from build123d import *

# Parameters (mm, degrees)
F0_W     = 40
F0_H     = 10
F1_DEPTH = 5
F3_DEPTH = 2.5
F4_R     = 3.5
F5_DEPTH = 7.501
F6_W     = 36.25
F6_H     = 7
F7_DEPTH = 7.501


with BuildPart() as f1:
    # F0 (on Top) → F1 (new body)
    with BuildSketch(Plane.XY):
        with Locations((20, 5)):
            Rectangle(F0_W, F0_H)
    extrude(amount=F1_DEPTH)

    # F2 (on face) → F3 (join)
    with BuildSketch(Plane.XY.offset(5)):
        with BuildLine():
            Line((40, 0), (45, 0))
            ThreePointArc((45, 0), (50, 5), (45, 10))
            Line((45, 10), (40, 10))
            Line((40, 10), (0, 10))
            Line((0, 10), (0, 0))
            Line((0, 0), (40, 0))
        make_face()
    extrude(amount=F3_DEPTH)

    # F4 (on face) → F5 (cut, through all)
    with BuildSketch(Plane.XY.offset(7.5)):
        with Locations((45, 5)):
            Circle(F4_R)
    extrude(amount=-F5_DEPTH, mode=Mode.SUBTRACT)

    # F6 (on face) → F7 (cut, through all)
    with BuildSketch(Plane.XY.offset(7.5)):
        with Locations((19.625, 5)):
            Rectangle(F6_W, F6_H)
    extrude(amount=-F7_DEPTH, mode=Mode.SUBTRACT)

    # F8: F1 across plane


with BuildPart() as f1_1:
    add(f1.part)
    add(f1.part.mirror(Plane.XY))


solid = f1_1.part
Geometry: final body of the model. Coordinates: model frame, mm. A direction names the side the tool comes from. Coordinates: 2 decimals unless noted, no trailing zeros. Order: outer loops, then holes, each group sorted by start corner. A loop starts at its lowest first (then second) coordinate and runs counter-clockwise, first axis right, second up. Notation, with made-up numbers: M 56,15.5 L 111,15.5 A9 cw 111,19.5 Z; hole C 21.25,77 d4. An arc over 180 degrees is marked long. One line per question, with ' | ' between items. Start each with the question number.
Item 1: Draft query along X for faces 1 (the flat face through (41.6, 7.3, -5)), 2 (the flat face through (37.75, 5, 0)), 3 (the flat face through (0, 5, 0)). Return one class per face: released by +X, released by -X, zero draft, split by the parting line, or undercut.
Item 2: Cut plane A-A, the plane z = -2. Return the cut outline in (x, y), then the cut area to 3 significant figures.
Item 3: Pin query (flat end, axial travel): pin 1 Ø5 at (y, z) = (8, -1.5) entering from +X. Return the tip coordinate at first contact, or that it passes through.
Item 4: Cut plane D-D, the plane z = 6.5. Return the cut outline in (x, y).
Item 5: Cut plane B-B, the plane y = 5. Return the cut outline in (x, z), then the cut area to 4 significant figures.
Item 6: Cut plane C-C, the plane x = 22. Return the cut outline in (y, z), then the cut area to 3 significant figures.
Item 7: Ray query, probe 1 along Y at (x, z) = (33, 2); probe 2 along X at (y, z) = (5.5, -2); probe 3 along Z at (x, y) = (40.5, 1.75). Return the intervals inside material, ascending. Write a range as [from, to].
Item 8: Set-up query: faces 4 (the flat face through (41.6, 7.3, 5)), 5 (the flat face through (27, 9, -7.5)), 6 (the flat face through (19, 1.5, 0)). Return all of +Z, -Z, +X, -X, +Y, -Y with unobstructed straight access to the full face (end or side cutting, diameter ignored); none if empty.
A:
1) face 1: zero draft | face 2: undercut | face 3: released by -X
2) outline: M 0,0 L 40,0 L 40,10 L 0,10 Z; hole M 1.5,1.5 L 37.75,1.5 L 37.75,8.5 L 1.5,8.5 Z | area: 146 mm2
3) pin 1: stops at x = 40
4) outline: M 0,0 L 45,0 A5 ccw 45,10 L 0,10 Z; hole M 1.5,1.5 L 37.75,1.5 L 37.75,8.5 L 1.5,8.5 Z; hole C 45,5 d7
5) outline: M 0,-7.5 L 1.5,-7.5 L 1.5,7.5 L 0,7.5 Z; M 37.75,-7.5 L 41.5,-7.5 L 41.5,-5 L 40,-5 L 40,5 L 41.5,5 L 41.5,7.5 L 37.75,7.5 Z; M 48.5,-7.5 L 50,-7.5 L 50,-5 L 48.5,-5 Z; M 48.5,5 L 50,5 L 50,7.5 L 48.5,7.5 Z | area: 71.25 mm2
6) outline: M 0,-7.5 L 1.5,-7.5 L 1.5,7.5 L 0,7.5 Z; M 8.5,-7.5 L 10,-7.5 L 10,7.5 L 8.5,7.5 Z | area: 45.0 mm2
7) probe 1: y = [0, 1.5], [8.5, 10] | probe 2: x = [0, 1.5], [37.75, 40] | probe 3: z = [-7.5, -5], [5, 7.5]
8) face 4: +X, +Y, -Y | face 5: -Z, +X, -X, +Y, -Y | face 6: +Z, -Z
